```python
from build123d import *

# Parameters (mm, degrees)
SKETCH1_R           = 20
SKETCH1_R_2         = 1.55
BOSS_EXTRUDE1_DEPTH = 3
BOSS_EXTRUDE2_DEPTH = 20


with BuildPart() as part:
    # Sketch1 → Boss-Extrude1 (new body)
    # profile 1 of 2: a face of its own
    with BuildSketch(Plane.XY):
        Circle(SKETCH1_R)
        with Locations((-10.606601718, -10.606601718)):
            Circle(SKETCH1_R_2, mode=Mode.SUBTRACT)
        with Locations((10.606601718, -10.606601718)):
            Circle(SKETCH1_R_2, mode=Mode.SUBTRACT)
        with Locations((-10.606601718, 10.606601718)):
            Circle(SKETCH1_R_2, mode=Mode.SUBTRACT)
        with BuildLine():
            ThreePointArc((4.125, 0), (-1.684302549, -3.765468088), (-2.749545417, 3.075))
            ThreePointArc((-2.749545417, 3.075), (0, 4.125), (2.749545417, 3.075))
            ThreePointArc((2.749545417, 3.075), (3.765468088, 1.684302549), (4.125, 0))
        make_face(mode=Mode.SUBTRACT)
        with Locations((10.606601718, 10.606601718)):
            Circle(SKETCH1_R_2, mode=Mode.SUBTRACT)
    # profile 2 of 2: a face of its own
    with BuildSketch(Plane.XY):
        with BuildLine():
            ThreePointArc((2.749545417, 3.075), (0, 4.125), (-2.749545417, 3.075))
            Line((-2.749545417, 3.075), (2.749545417, 3.075))
        make_face()
    extrude(amount=BOSS_EXTRUDE1_DEPTH)

    # Sketch1_3 → Boss-Extrude2 (add)
    with BuildSketch(Plane.XY):
        with BuildLine():
            Line((2.749545417, 3.075), (-2.749545417, 3.075))
            ThreePointArc((-2.749545417, 3.075), (-1.684302549, -3.765468088), (4.125, 0))
            ThreePointArc((4.125, 0), (3.765468088, 1.684302549), (2.749545417, 3.075))
        make_face()
    extrude(amount=BOSS_EXTRUDE2_DEPTH)


solid = part.part
```
Work out the finished part from the listing and answer in its coordinate system (mm). A direction names the side the tool comes from. Coordinates: 2 decimals unless noted, no trailing zeros. Write each loop counter-clockwise with the first axis right and the second up, starting at its lowest first coordinate (ties: lowest second). Pieces come first, ordered by that corner, then holes.
Q1. Determine the mould class of faces 1 (the face through (-4.336, -19.524, 1.479)), 2 (the face through (9.06, -10.54, 1.48)), 3 (the face through (9.38, 9.66, 1.48)), 4 (the face through (0, 0, 20)) for opening direction X: released by +X, released by -X, zero draft, split by the parting line, or undercut.
Q2. Which of the six approach directions +Z, -Z, +X, -X, +Y, -Y give full straight-line access (tool end or side, diameter ignored) to faces 5 (the face through (0, 0, 0)), 6 (the face through (0, 3.075, 11))?
Q3. Each of these flat-tipped pins is pushed along its axis until it touches: pin 1 Ø2.5 at (x, y) = (10.61, -10.61) entering from -Z; pin 2 Ø1 at (y, z) = (1, 17.5) entering from -X; pin 3 Ø6 at (y, z) = (0, 9) entering from +X (3 decimals); pin 4 Ø1.5 at (y, z) = (2.5, 12.5) entering from -X. Where does it stop, or does it pass through?
Q4. Find the intervals of material crossed by line 1 (Z direction, x = -13.5, y = 4); line 2 (X direction, y = 3, z = 2.5); line 3 (Y direction, x = -4, z = 1.5), in increasing order.
Q5. A cutting plane is placed at D-D, the plane y = 2. Give the vertices of the cut face in (x, z).
Q6. A cutting plane is placed at A-A, the plane y = 10. Give the vertices of the cut face in (x, z).
Q7. A cutting plane is placed at B-B, the plane z = 1.5. Give the vertices of the cut face in (x, y), then the cut area to 3 significant figures.
Q8. A cutting plane is placed at C-C, the plane x = 0. Give the vertices of the cut face in (y, z) (3 decimals), then the cut area to 3 significant figures.
Findings below:
1. face 1: split by the parting line
1. face 2: undercut
1. face 3: undercut
1. face 4: zero draft
2. face 5: -Z, +X, -X, +Y, -Y
2. face 6: +Z, +X, -X, +Y
3. pin 1: passes through
3. pin 2: stops at x = -4.09
3. pin 3: stops at x = 4.125
3. pin 4: stops at x = -3.74
4. line 1: z = 0 to 3
4. line 2: x = -19.77 to 19.77
4. line 3: y = -19.6 to 19.6
5. outline: (-19.9, 0) - (19.9, 0) - (19.9, 3) - (3.61, 3) - (3.61, 20) - (-3.61, 20) - (-3.61, 3) - (-19.9, 3) - close
6. outline: (-17.32, 0) - (-12.03, 0) - (-12.03, 3) - (-17.32, 3) - close; (-9.18, 0) - (9.18, 0) - (9.18, 3) - (-9.18, 3) - close; (12.03, 0) - (17.32, 0) - (17.32, 3) - (12.03, 3) - close
7. outline: circle Ø40 at (0, 0); hole circle Ø3.1 at (-10.61, -10.61); hole circle Ø3.1 at (-10.61, 10.61); hole circle Ø3.1 at (10.61, -10.61); hole circle Ø3.1 at (10.61, 10.61)
7. area: 1,230 mm2
8. outline: (-20, 0) - (20, 0) - (20, 3) - (3.075, 3) - (3.075, 20) - (-4.125, 20) - (-4.125, 3) - (-20, 3) - close
8. area: 242 mm2
